Source: CAD feature listing. Evaluate the final solid. Frame: model axes, mm. Round coordinates to 2 decimals unless told otherwise and drop trailing zeros. Loops run counter-clockwise (first coordinate to the right, second up) from the corner with the lowest first, then second, coordinate; pieces in that order, holes last.
(1) Section B-B, the plane y = 98.5. Return the cut outline in (x, z), plus the area to 3 significant figures.
(2) Section D-D, the plane x = -46.5. Return the cut outline in (y, z).
(3) First-contact query: pin 1 Ø3.5 at (x, y) = (0, 78.5) entering from -Z; pin 2 Ø5.5 at (x, y) = (46, 8.5) entering from -Z; pin 3 Ø1 at (x, z) = (-46, 1.5) entering from +Y. Flat tips, straight axial feed; report the tip coordinate or a pass-through.
(4) Section A-A, the plane y = 13.5. Return the cut outline in (x, z), plus the area to 3 significant figures.
(5) Section C-C, the plane x = 0. Return the cut outline in (y, z), plus the area to 3 significant figures.
(6) Material intervals for probe 1 along Y at (x, z) = (0, 0.5); probe 2 along X at (y, z) = (-32.5, 0.8); probe 3 along Y at (x, z) = (-32.5, 1.9), sorted ascending.
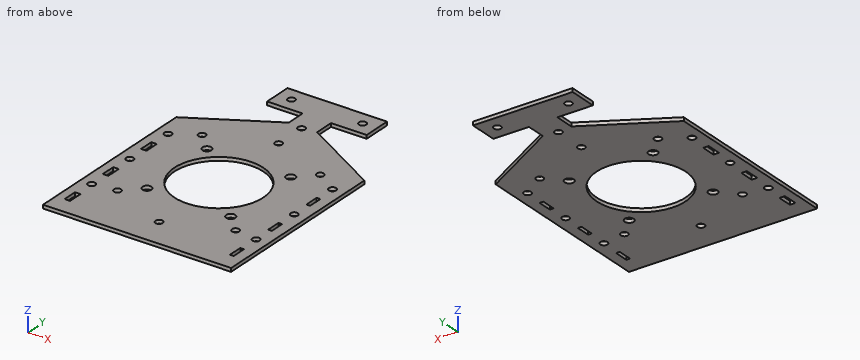
```python
from build123d import *

# Parameters (mm, degrees)
SKETCH_1_R      = 2.55
SKETCH_1_R_2    = 25
SKETCH_1_R_3    = 2.05
SKETCH_1_W      = 2.1
SKETCH_1_H      = 8.1
SKETCH_1_W_2    = 3.1
EXTRUDE_1_DEPTH = 2


with BuildPart() as part:
    # 草图1 → 凸台-拉伸1 (new body)
    with BuildSketch(Plane.XY):
        Polygon((-52.9, 53.883164809), (-52.9, -50.790000001), (52.9, -50.790000001), (52.9, 53.883164809), (8, 79.569735886), (8, 90.5), (28, 90.5), (28, 106.5), (-28, 106.5), (-28, 90.5), (-8, 90.5), (-8, 79.569735886), align=None)
        with Locations((-23.57, 37.07)):
            Circle(SKETCH_1_R, mode=Mode.SUBTRACT)
        with Locations((-23.57, -10.07)):
            Circle(SKETCH_1_R, mode=Mode.SUBTRACT)
        with Locations((23.57, -10.07)):
            Circle(SKETCH_1_R, mode=Mode.SUBTRACT)
        with Locations((23.57, 37.07)):
            Circle(SKETCH_1_R, mode=Mode.SUBTRACT)
        with Locations((0, 13.5)):
            Circle(SKETCH_1_R_2, mode=Mode.SUBTRACT)
        with Locations((0, 60.5)):
            Circle(SKETCH_1_R_3, mode=Mode.SUBTRACT)
        with Locations((33.234018716, 46.734018716)):
            Circle(SKETCH_1_R_3, mode=Mode.SUBTRACT)
        with Locations((33.234018716, -19.734018716)):
            Circle(SKETCH_1_R_3, mode=Mode.SUBTRACT)
        with Locations((0, -33.5)):
            Circle(SKETCH_1_R_3, mode=Mode.SUBTRACT)
        with Locations((-33.234018716, -19.734018716)):
            Circle(SKETCH_1_R_3, mode=Mode.SUBTRACT)
        with Locations((-33.234018716, 46.734018716)):
            Circle(SKETCH_1_R_3, mode=Mode.SUBTRACT)
        with Locations((0, 78.5)):
            Circle(SKETCH_1_R_3, mode=Mode.SUBTRACT)
        with Locations((-20, 98.5)):
            Circle(SKETCH_1_R_3, mode=Mode.SUBTRACT)
        with Locations((20, 98.5)):
            Circle(SKETCH_1_R_3, mode=Mode.SUBTRACT)
        with Locations((46, 8.5)):
            Circle(SKETCH_1_R_3, mode=Mode.SUBTRACT)
        with Locations((46, -21.5)):
            Circle(SKETCH_1_R_3, mode=Mode.SUBTRACT)
        with Locations((46, 38.5)):
            Circle(SKETCH_1_R_3, mode=Mode.SUBTRACT)
        with Locations((-46.5, -21.5)):
            Circle(SKETCH_1_R_3, mode=Mode.SUBTRACT)
        with Locations((-46.5, 8.5)):
            Circle(SKETCH_1_R_3, mode=Mode.SUBTRACT)
        with Locations((-46.5, 38.5)):
            Circle(SKETCH_1_R_3, mode=Mode.SUBTRACT)
        with Locations((46, 23.5)):
            Rectangle(SKETCH_1_W, SKETCH_1_H, mode=Mode.SUBTRACT)
        with Locations((46, -6.5)):
            Rectangle(SKETCH_1_W, SKETCH_1_H, mode=Mode.SUBTRACT)
        with Locations((46, -36.5)):
            Rectangle(SKETCH_1_W, SKETCH_1_H, mode=Mode.SUBTRACT)
        with Locations((-46.5, 23.5)):
            Rectangle(SKETCH_1_W_2, SKETCH_1_H, mode=Mode.SUBTRACT)
        with Locations((-46.5, -6.5)):
            Rectangle(SKETCH_1_W_2, SKETCH_1_H, mode=Mode.SUBTRACT)
        with Locations((-46.5, -36.5)):
            Rectangle(SKETCH_1_W_2, SKETCH_1_H, mode=Mode.SUBTRACT)
    extrude(amount=EXTRUDE_1_DEPTH)


solid = part.part
```
Output values:
1. outline: (-28, 0) - (-22.05, 0) - (-22.05, 2) - (-28, 2) - close; (-17.95, 0) - (17.95, 0) - (17.95, 2) - (-17.95, 2) - close; (22.05, 0) - (28, 0) - (28, 2) - (22.05, 2) - close
1. area: 95.6 mm2
2. outline: (-50.79, 0) - (-40.55, 0) - (-40.55, 2) - (-50.79, 2) - close; (-32.45, 0) - (-23.55, 0) - (-23.55, 2) - (-32.45, 2) - close; (-19.45, 0) - (-10.55, 0) - (-10.55, 2) - (-19.45, 2) - close; (-2.45, 0) - (6.45, 0) - (6.45, 2) - (-2.45, 2) - close; (10.55, 0) - (19.45, 0) - (19.45, 2) - (10.55, 2) - close; (27.55, 0) - (36.45, 0) - (36.45, 2) - (27.55, 2) - close; (40.55, 0) - (57.54, 0) - (57.54, 2) - (40.55, 2) - close
3. pin 1: passes through
3. pin 2: stops at z = 0
3. pin 3: stops at y = 58.12
4. outline: (-52.9, 0) - (-25, 0) - (-25, 2) - (-52.9, 2) - close; (25, 0) - (52.9, 0) - (52.9, 2) - (25, 2) - close
4. area: 112 mm2
5. outline: (-50.79, 0) - (-35.55, 0) - (-35.55, 2) - (-50.79, 2) - close; (-31.45, 0) - (-11.5, 0) - (-11.5, 2) - (-31.45, 2) - close; (38.5, 0) - (58.45, 0) - (58.45, 2) - (38.5, 2) - close; (62.55, 0) - (76.45, 0) - (76.45, 2) - (62.55, 2) - close; (80.55, 0) - (106.5, 0) - (106.5, 2) - (80.55, 2) - close
5. area: 190 mm2
6. probe 1: y = -50.79 to -35.55, -31.45 to -11.5, 38.5 to 58.45, 62.55 to 76.45, 80.55 to 106.5
6. probe 2: x = -52.9 to -48.05, -44.95 to -1.79, 1.79 to 44.95, 47.05 to 52.9
6. probe 3: y = -50.79 to -21.65, -17.82 to 44.82, 48.65 to 65.55
